```python
from build123d import *

# Parameters (mm, degrees)
SKETCH1_R               = 20
BOSS_EXTRUDE1_DEPTH     = 15
CUT_EXTRUDE1_DEPTH      = 1
CUT_EXTRUDE1_DEPTH_BACK = 5
SKETCH3_R               = 3.5
CUT_EXTRUDE2_DEPTH      = 11
SKETCH5_R               = 7.5
CUT_EXTRUDE4_DEPTH      = 5
SKETCH4_R               = 6
CUT_EXTRUDE5_DEPTH      = 16
CUT_EXTRUDE6_DEPTH      = 1
CUT_EXTRUDE6_DEPTH_BACK = 16
CUT_EXTRUDE7_DEPTH      = 1
CUT_EXTRUDE7_DEPTH_BACK = 16


with BuildPart() as part:
    # Sketch1 → Boss-Extrude1 (new body)
    with BuildSketch(Plane(origin=(0, 0, 0), x_dir=(1, 0, 0), z_dir=(0, 1, 0))):
        Circle(SKETCH1_R)
    extrude(amount=BOSS_EXTRUDE1_DEPTH)

    # Sketch2 → Cut-Extrude1 (cut, two sides)
    with BuildSketch(Plane(origin=(0, 15, 0), x_dir=(1, 0, 0), z_dir=(0, 1, 0))) as cut_extrude1_sk:
        Polygon((4.074284854, 123.342943671), (10.2938366, 17.14750501), (12.225151258, -15.828634708), (18.444703004, -122.024073369), (230.835580327, -109.584969878), (216.465162177, 135.782047162), align=None)
    extrude(amount=CUT_EXTRUDE1_DEPTH, mode=Mode.SUBTRACT)
    extrude(cut_extrude1_sk.sketch, amount=-CUT_EXTRUDE1_DEPTH_BACK, mode=Mode.SUBTRACT)

    # Sketch3 → Cut-Extrude2 (cut, through all)
    with BuildSketch(Plane(origin=(0, 10, 0), x_dir=(1, 0, 0), z_dir=(0, 1, 0))):
        with Locations((15.014261177, 2.902690148)):
            Circle(SKETCH3_R)
    extrude(amount=-CUT_EXTRUDE2_DEPTH, mode=Mode.SUBTRACT)

    # Sketch5 → Cut-Extrude4 (cut)
    with BuildSketch(Plane(origin=(0, 15, 0), x_dir=(1, 0, 0), z_dir=(0, 1, 0))):
        with Locations((-9.188292451, 1.230126279)):
            Circle(SKETCH5_R)
    extrude(amount=-CUT_EXTRUDE4_DEPTH, mode=Mode.SUBTRACT)

    # Sketch4 → Cut-Extrude5 (cut, through all)
    with BuildSketch(Plane(origin=(0, 15, 0), x_dir=(1, 0, 0), z_dir=(0, 1, 0))):
        with Locations((-9.188292451, 1.230126279)):
            Circle(SKETCH4_R)
    extrude(amount=-CUT_EXTRUDE5_DEPTH, mode=Mode.SUBTRACT)

    # Sketch6 → Cut-Extrude6 (cut, two sides)
    with BuildSketch(Plane(origin=(0, 15, 0), x_dir=(1, 0, 0), z_dir=(0, 1, 0))) as cut_extrude6_sk:
        Polygon((-122.787131769, -18.599673993), (-17.584679199, -9.527804442), (8.38493326, -7.288380068), (9.284012328, -17.714601748), (18.355881879, -122.917054318), (-107.166589312, -292.750880754), (-248.30960296, -188.433500429), align=None)
    extrude(amount=CUT_EXTRUDE6_DEPTH, mode=Mode.SUBTRACT)
    extrude(cut_extrude6_sk.sketch, amount=-CUT_EXTRUDE6_DEPTH_BACK, mode=Mode.SUBTRACT)

    # Sketch7 → Cut-Extrude7 (cut, two sides)
    with BuildSketch(Plane(origin=(0, 15, 0), x_dir=(1, 0, 0), z_dir=(0, 1, 0))) as cut_extrude7_sk:
        Polygon((-119.21548429, -0.03712377), (-16.591552302, 11.167828446), (7.395972386, 13.786896559), (6.849658032, 18.79048123), (-4.355294184, 121.414413217), (-154.363796188, 263.281741412), (-269.223986293, 141.830204426), align=None)
    extrude(amount=CUT_EXTRUDE7_DEPTH, mode=Mode.SUBTRACT)
    extrude(cut_extrude7_sk.sketch, amount=-CUT_EXTRUDE7_DEPTH_BACK, mode=Mode.SUBTRACT)


solid = part.part
```
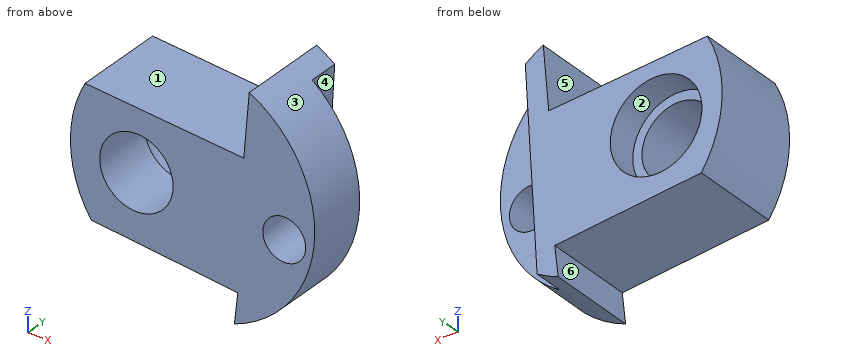
For this review, take the finished solid that the model builds, in its own axes (mm). Face numbers are marked on the shaded views. A direction names the side the tool comes from. Round coordinates to 2 decimals unless told otherwise and drop trailing zeros. Loops run counter-clockwise (first coordinate to the right, second up) from the corner with the lowest first, then second, coordinate; pieces in that order, holes last.
Q1. Insertion check: pin 1 Ø8 at (x, y) = (-14.5, 13) entering from +Z; pin 2 Ø10.5 at (x, z) = (17, 5.5) entering from +Y; pin 3 Ø5 at (x, z) = (-11.5, -1) entering from -Y; pin 4 Ø4 at (x, y) = (11, 2) entering from -Z. Each pin has a flat end and moves straight along its axis. Give the tip position at first contact, or say it passes through.
Result sheet:
pin 1: stops at z = 9.53
pin 2: stops at y = 10
pin 3: passes through
pin 4: stops at z = -17.86
Q2. To check wall thickness, follow line 1 along X through (y, z) = (1, -2); line 2 along X through (y, z) = (0.5, -6); line 3 along Z through (x, y) = (-14, 13). State the ranges of each line that lie inside material, in increasing order.
Result sheet:
line 1: x = -19.9 to -15.14, -3.24 to 11.63, 18.4 to 19.9
line 2: x = -19.08 to -12.83, -5.55 to 13.38, 16.64 to 19.08
line 3: z = -11.45 to -6.98, 4.52 to 9.22
Q3. Add section D-D on x = -6. Write out the cut boundary in (y, z), plus the area to 3 significant figures.
Result sheet:
outline: (0, -12.32) - (15, -12.32) - (15, -8.02) - (10, -8.02) - (10, -6.31) - (0, -6.31) - close; (0, 3.85) - (10, 3.85) - (10, 5.56) - (15, 5.56) - (15, 8.53) - (0, 8.53) - close
area: 143 mm2
Q4. Add section C-C on y = 9. Write out the cut boundary in (x, z).
Result sheet:
outline: (-17.58, 9.53) arc R20 ccw to (-16.59, -11.17) - (7.4, -13.79) - (6.85, -18.79) arc R20 ccw to (9.28, 17.71) - (8.38, 7.29) - close; hole circle Ø12 at (-9.19, -1.23); hole circle Ø7 at (15.01, -2.9)
Q5. Add section A-A on x = -14. Write out the cut boundary in (y, z), plus the area to 3 significant figures.
Result sheet:
outline: (0, -11.45) - (15, -11.45) - (15, -6.98) - (10, -6.98) - (10, -4.81) - (0, -4.81) - close; (0, 2.35) - (10, 2.35) - (10, 4.52) - (15, 4.52) - (15, 9.22) - (0, 9.22) - close
area: 181 mm2
Q6. Machinability: for the marked faces 4, 5 and 6, which of the approach directions +Z, -Z, +X, -X, +Y, -Y give a long, thin tool a straight path to every point of the face, cutting with its end or side? Answer none if there is none.
Result sheet:
face 4: -Z, +X, +Y
face 5: +Z, +Y, -Y
face 6: -X, +Y, -Y
Q7. Add section B-B on z = 0. Write out the cut boundary in (x, y), plus the area to 3 significant figures.
Result sheet:
outline: (-20, 0) - (-15.06, 0) - (-15.06, 10) - (-16.59, 10) - (-16.59, 15) - (-20, 15) - close; (-3.32, 0) - (13.06, 0) - (13.06, 10) - (11.3, 10) - (11.3, 15) - (-1.79, 15) - (-1.79, 10) - (-3.32, 10) - close; (16.97, 0) - (20, 0) - (20, 10) - (16.97, 10) - close
area: 326 mm2
Q8. Mouldability with a two-part tool opening along Z and no side actions: class the marked faces 1, 2 and 3 as +Z half, -Z half, draft (parallel to the pull), parting line (faces both ways), or undercut.
Result sheet:
face 1: +Z half
face 2: undercut
face 3: parting line
